```python
from build123d import *

# Parameters (mm, degrees)
BOSS_EXTRUDE1_DEPTH = 6.35
SKETCH4_R           = 2.75
CUT_EXTRUDE1_DEPTH  = 10
SKETCH5_R           = 2.75
CUT_EXTRUDE2_DEPTH  = 94.06622642
FILLET1_R           = 40
FILLET2_R           = 2


with BuildPart() as part:
    # Sketch2 → Boss-Extrude1 (new body)
    with BuildSketch(Plane.XY):
        Polygon((0, 0), (20, 0), (20, 31), (61, 31), (61, 70), (0, 70), align=None)
    extrude(amount=BOSS_EXTRUDE1_DEPTH)

    # Sketch4 → Cut-Extrude1 (cut)
    with BuildSketch(Plane(origin=(0, 0, 0), x_dir=(-1, 0, 0), z_dir=(0, 0, -1))):
        with Locations((-26, 64)):
            Circle(SKETCH4_R)
        with Locations((-54.999998701, 64)):
            Circle(SKETCH4_R)
        with Locations((-55, 37)):
            Circle(SKETCH4_R)
        with Locations((-26.000001299, 37)):
            Circle(SKETCH4_R)
    extrude(amount=-CUT_EXTRUDE1_DEPTH, mode=Mode.SUBTRACT)

    # Sketch5 → Cut-Extrude2 (cut, through all)
    with BuildSketch(Plane.XY.offset(6.35)):
        with Locations((10, 8)):
            Circle(SKETCH5_R)
        with Locations((10, 26)):
            Circle(SKETCH5_R)
        with Locations((10, 44)):
            Circle(SKETCH5_R)
        with Locations((10, 62)):
            Circle(SKETCH5_R)
    extrude(amount=-CUT_EXTRUDE2_DEPTH, mode=Mode.SUBTRACT)

    # Fillet1
    # the kernel refuses this fillet: 40 mm, written as the material it adds along each edge
    with BuildSketch(Plane(origin=(20, 31, 0), x_dir=(0, -1, 0), z_dir=(0, 0, 1))) as fillet1_piece_1:
        with BuildLine():
            CenterArc((40, 38.97435054), FILLET1_R, 180, 76.997121837)
            Line((0, 38.97435054), (-0.8, 38.97435054))
            Line((-0.8, 38.97435054), (-0.8, 0))
            Line((-0.8, 0), (0, -0.8))
            ThreePointArc((0, -0.8), (15.5, -0.8), (30.82, -0.779487011))
            Line((30.82, -0.779487011), (31, 0))
        make_face()
    extrude(amount=6.35)

    # Fillet2
    fillet2_edges = [part.edges().sort_by_distance(p)[0] for p in [
        (0, 70, 3.175),
        (61, 70, 3.175),
        (61, 31, 3.175),
        (20, 0, 3.175),
        (0, 0, 3.175),
    ]]
    fillet(fillet2_edges, radius=FILLET2_R)


solid = part.part
```
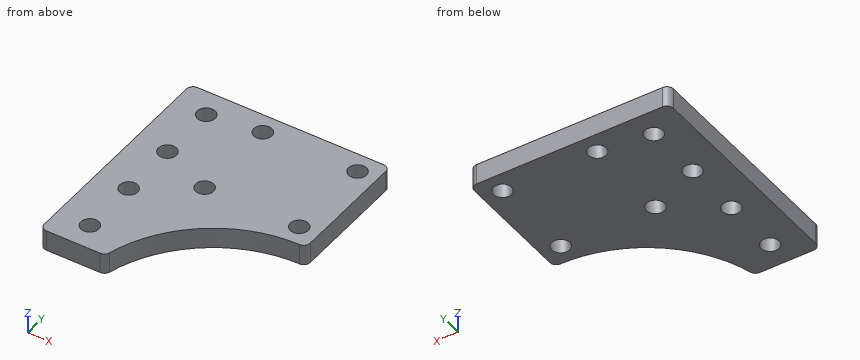
Geometry check sheet. Reference: the model listing, model coordinates, mm. Give positions to 0.01 mm unless a question says otherwise; leave off trailing zeros. Order: outer loops, then holes, each group sorted by start corner. A loop starts at its lowest first (then second) coordinate and runs counter-clockwise, first axis right, second up. Notation, with made-up numbers: (2, -38) -> (59, -38) arc R17 ccw to (59, -34) -> close; hole circle Ø4 at (-17, -23.75). An arc over 180 degrees is marked (long way). Write each question's results on one line, items separated by ' | '. Start each with the question number.
(1) Sectioned sample at D-D (y = 64). Enter the section's corners in (x, z).
(2) Gauge pin test, flat ends, axial feed: P1, Ø1.5, axis at y = 31.5, z = 5.5, coming from the +X side; P2, Ø3, axis at x = 51, z = 3, coming from the -Y side. Record the tip position at first contact, or that the pin passes through.
(3) Sectioned sample at A-A (x = 10). Enter the section's corners in (y, z).
(4) Sectioned sample at C-C (y = 37). Enter the section's corners in (x, z).
(5) Sectioned sample at B-B (z = 2.75). Give the number of separate pieces and of enclosed holes in the cut face, plus the area to 3 significant figures.
(6) Scan lines: line 1 (Y direction, x = 10, z = 4.5); line 2 (Y direction, x = 26, z = 1.5); line 3 (X direction, y = 38, z = 1.75). Record each from-to range of solid material in increasing order.
Answer below:
1) outline: (0, 0) -> (8.11, 0) -> (8.11, 6.35) -> (0, 6.35) -> close; (11.89, 0) -> (23.25, 0) -> (23.25, 6.35) -> (11.89, 6.35) -> close; (28.75, 0) -> (52.25, 0) -> (52.25, 6.35) -> (28.75, 6.35) -> close; (57.75, 0) -> (61, 0) -> (61, 6.35) -> (57.75, 6.35) -> close
2) P1: x = 60.85 | P2: y = 29.86
3) outline: (0, 0) -> (5.25, 0) -> (5.25, 6.35) -> (0, 6.35) -> close; (10.75, 0) -> (23.25, 0) -> (23.25, 6.35) -> (10.75, 6.35) -> close; (28.75, 0) -> (41.25, 0) -> (41.25, 6.35) -> (28.75, 6.35) -> close; (46.75, 0) -> (59.25, 0) -> (59.25, 6.35) -> (46.75, 6.35) -> close; (64.75, 0) -> (70, 0) -> (70, 6.35) -> (64.75, 6.35) -> close
4) outline: (0, 0) -> (23.25, 0) -> (23.25, 6.35) -> (0, 6.35) -> close; (28.75, 0) -> (52.25, 0) -> (52.25, 6.35) -> (28.75, 6.35) -> close; (57.75, 0) -> (61, 0) -> (61, 6.35) -> (57.75, 6.35) -> close
5) separate pieces: 1 | enclosed holes: 8 | area: 3,110 mm2
6) line 1: 0 to 5.25, 10.75 to 23.25, 28.75 to 41.25, 46.75 to 59.25, 64.75 to 70 | line 2: 13.64 to 34.25, 39.75 to 61.25, 66.75 to 70 | line 3: 0 to 23.44, 28.56 to 52.44, 57.56 to 61
